```python
from build123d import *

# Parameters (mm, degrees)
F0_W        = 762
F0_H        = 203.2
F1_DEPTH    = 76.2
F2_R        = 101.59999
F3_W        = 643.4846520424
F3_H        = 146.4012786746
F4_DEPTH    = 63.5
F5_T1_DEPTH = 63.5
F8_DEPTH    = 25.4
F9_R        = 7.62
F10_DEPTH   = 25.4


# Not quite as in the source:
# - a fillet or chamfer that OpenCascade refuses, or shapes differently, is made with other operations: its cross-section is extruded or revolved along the edge and cut away or added
# - a fillet or chamfer is up to 0.001 mm smaller than in the source, because OpenCascade refuses the exact size


with BuildPart() as f1:
    # F0 (on Right) → F1 (new body)
    with BuildSketch(Plane.YZ):
        with Locations((20.2849134803, -13.820597699)):
            Rectangle(F0_W, F0_H)
    extrude(amount=F1_DEPTH)

    # F2 (radius 101.6 in the source; OpenCascade refuses exactly that, so slightly less here)
    f2_edges = [f1.edges().sort_by_distance(p)[0] for p in [
        (38.1, -360.715087, 87.779402),
        (38.1, -360.715087, -115.420598),
        (38.1, 401.284913, 87.779402),
        (38.1, 401.284913, -115.420598),
    ]]
    fillet(f2_edges, radius=F2_R)

    # F3 (on face) → F4 (cut)
    with BuildSketch(Plane.YZ.offset(76.2)):
        with Locations((24.1151750088, -15.0973536074)):
            Rectangle(F3_W, F3_H)
    extrude(amount=-F4_DEPTH, mode=Mode.SUBTRACT)

    # F5: fillet of radius 76.2 on 4 edges, made by hand

    # F5_s2 → F5_t1 (join)
    with BuildSketch(Plane.YZ.offset(12.7)):
        with BuildLine():
            ThreePointArc((-221.4271510124, 58.1032857299), (-275.3086877388, 35.7848224563), (-297.6271510124, -18.0967142701))
            Line((-297.6271510124, -18.0967142701), (-297.6271510124, 58.1032857299))
            Line((-297.6271510124, 58.1032857299), (-221.4271510124, 58.1032857299))
        make_face()
        with BuildLine():
            ThreePointArc((-297.6271510124, -12.0979929447), (-275.3086877388, -65.9795296711), (-221.4271510124, -88.2979929447))
            Line((-221.4271510124, -88.2979929447), (-297.6271510124, -88.2979929447))
            Line((-297.6271510124, -88.2979929447), (-297.6271510124, -12.0979929447))
        make_face()
        with BuildLine():
            ThreePointArc((269.65750103, 58.1032857299), (323.5390377564, 35.7848224563), (345.85750103, -18.0967142701))
            Line((345.85750103, -18.0967142701), (345.85750103, 58.1032857299))
            Line((345.85750103, 58.1032857299), (269.65750103, 58.1032857299))
        make_face()
        with BuildLine():
            ThreePointArc((269.65750103, -88.2979929447), (323.5390377564, -65.9795296711), (345.85750103, -12.0979929447))
            Line((345.85750103, -12.0979929447), (345.85750103, -88.2979929447))
            Line((345.85750103, -88.2979929447), (269.65750103, -88.2979929447))
        make_face()
    extrude(amount=F5_T1_DEPTH)

    # F7 (on face) → F8 (cut)
    with BuildSketch(Plane(origin=(0, 0, 0), x_dir=(0, -1, 0), z_dir=(-1, 0, 0))):
        with BuildLine():
            ThreePointArc((-276.6019562226, -21.4793750917), (-268.0456280954, -25.6827990477), (-262.0824047375, -18.2450916618))
            ThreePointArc((-262.0824047375, -18.2450916618), (-262.2195694481, -16.8057946003), (-262.6261254806, -15.4183140124))
            ThreePointArc((-262.6261254806, -15.4183140124), (-272.557495484, -11.6617121999), (-276.6019562226, -21.4793750917))
        make_face()
    extrude(amount=-F8_DEPTH, mode=Mode.SUBTRACT)

    # F9 (on face) → F10 (cut)
    with BuildSketch(Plane(origin=(0, 0, 0), x_dir=(0, -1, 0), z_dir=(-1, 0, 0))):
        with Locations((221.1862802505, -18.3496363461)):
            Circle(F9_R)
    extrude(amount=-F10_DEPTH, mode=Mode.SUBTRACT)


solid = f1.part
```
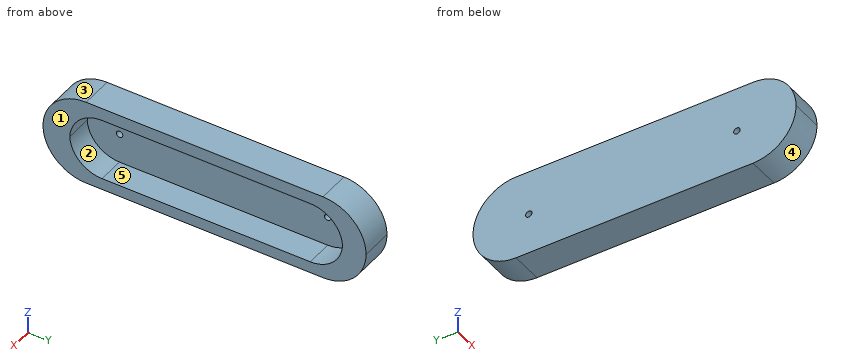
Verification items for the finished model (mm, model axes). Face numbers are marked on the shaded views. A direction names the side the tool comes from. Coordinates: 2 decimals unless noted, no trailing zeros. Loops run counter-clockwise (first coordinate to the right, second up) from the corner with the lowest first, then second, coordinate; pieces in that order, holes last. Notation, with made-up numbers: (17.25, -38.5) - (40.25, -38.5) arc R22 ccw to (40.25, -5.5) - close; hole circle Ø9 at (-32.5, 23). An arc over 180 degrees is marked (long way). Put each result on its own line as item: value.
Item 1: Scan lines: line 1 along Y through (x, z) = (32.5, -15.5); line 2 along Z through (x, y) = (23, -224); line 3 along X through (y, z) = (54, -11.5). Record each from-to range of solid material in increasing order.
Conclusion:
line 1: y = -360.7 to -297.55, 345.78 to 401.27
line 2: z = -115.42 to -88.25, 58.06 to 87.78
line 3: x = 0 to 12.7
Item 2: Draft check along Z on the marked faces 1, 2 and 3. Enter one of: pulls with the +Z half, pulls with the -Z half, needs draft (parallel to the pull), parting line crosses it, or undercut.
Conclusion:
face 1: needs draft
face 2: undercut
face 3: pulls with the +Z half
Item 3: Set-up check for the marked faces 4 and 5: record each of +Z, -Z, +X, -X, +Y, -Y from which the full face is reachable in a straight line by a thin tool's end or side.
Conclusion:
face 4: -Z, +X, -X, -Y
face 5: +X
Item 4: Section check C-C (z = 3). Enter the section's corners in (x, y), then the cut area to 3 significant figures.
Conclusion:
outline: (0, -359.31) - (76.2, -359.31) - (76.2, -294.65) - (12.7, -294.65) - (12.7, 342.88) - (76.2, 342.88) - (76.2, 399.88) - (0, 399.88) - close
area: 17,400 mm2
Item 5: Section check B-B (y = -73). Enter the section's corners in (x, z).
Conclusion:
outline: (0, -115.42) - (76.2, -115.42) - (76.2, -88.3) - (12.7, -88.3) - (12.7, 58.1) - (76.2, 58.1) - (76.2, 87.78) - (0, 87.78) - close
Item 6: Gauge pin test, flat ends, axial feed: pin 1 Ø5 at (x, z) = (10.5, -86) entering from -Y; pin 2 Ø1 at (x, z) = (43.5, 13.5) entering from -Y; pin 3 Ø17.5 at (y, z) = (-221.19, -18.35) entering from +X. Record the tip position at first contact, or that the pin passes through.
Conclusion:
pin 1: stops at y = -333.06
pin 2: stops at y = -357.11
pin 3: stops at x = 12.7
